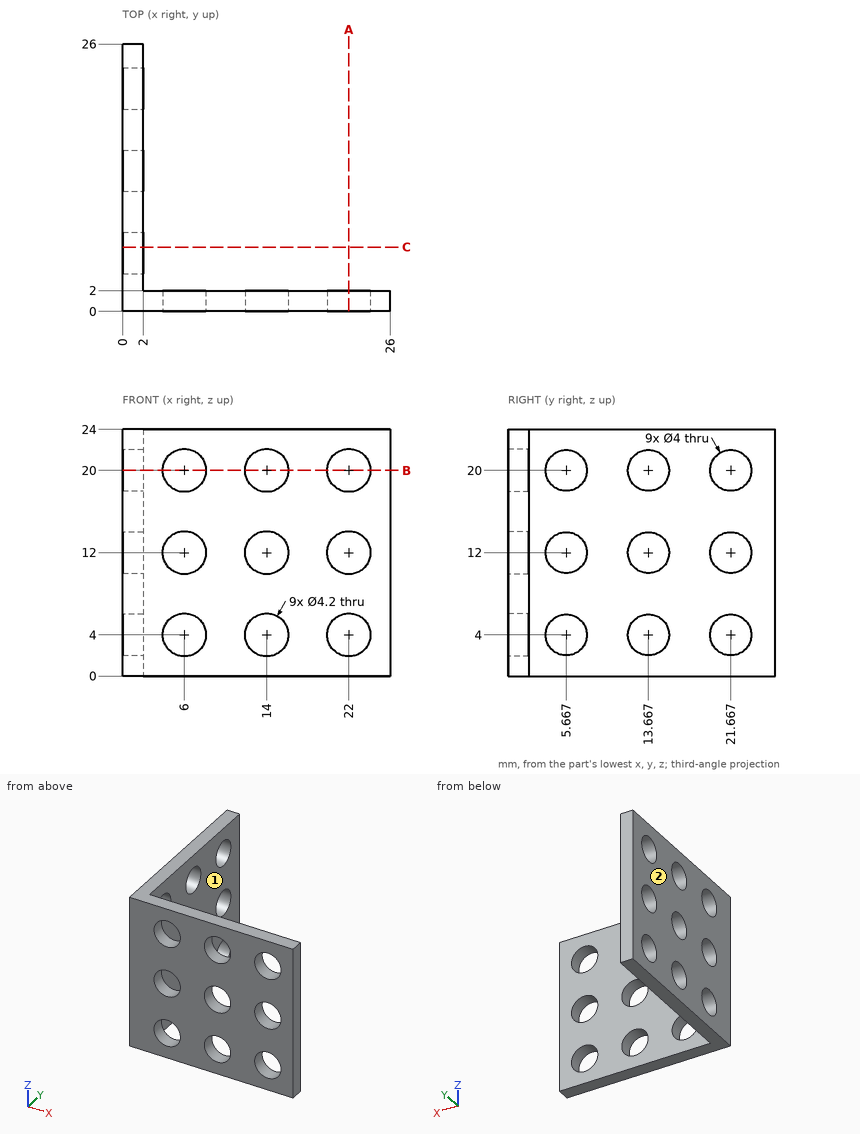
Part print with two shaded views. Sizes in mm from the minimum x, y, z corner. A direction names the side the tool comes from. Coordinates: 2 decimals unless noted, no trailing zeros. Loops run counter-clockwise (first coordinate to the right, second up) from the corner with the lowest first, then second, coordinate; pieces in that order, holes last. Notation, with made-up numbers: (-39.75, 68) -> (-1.75, 68) arc R35 cw to (-1.75, 102) -> close; hole circle Ø8 at (37.5, -18.5). An arc over 180 degrees is marked (long way). Answer as a JSON object with one key per item and string values.
Q1. Cut at A-A (x = 22). List the corners of the cut face in (y, z), and give its area (3 significant figures).
Report:
{"outline": "(0, 0) -> (2, 0) -> (2, 1.9) -> (0, 1.9) -> close; (0, 6.1) -> (2, 6.1) -> (2, 9.9) -> (0, 9.9) -> close; (0, 14.1) -> (2, 14.1) -> (2, 17.9) -> (0, 17.9) -> close; (0, 22.1) -> (2, 22.1) -> (2, 24) -> (0, 24) -> close", "area": "22.8 mm2"}
Q2. Flat gauge pins, fed straight in: P1, Ø4, axis at x = 6, z = 20, coming from the -Y side; P2, Ø5, axis at x = 8.5, z = 17, coming from the +Y side; P3, Ø5, axis at y = 21.67, z = 4, coming from the +X side. Where does each tip first touch, or does it go through?
Report:
{"P1": "passes through", "P2": "stops at y = 2", "P3": "stops at x = 2"}
Q3. Cut at B-B (z = 20). State how many separate pieces and enclosed holes the cut face has.
Report:
{"separate pieces": "7", "enclosed holes": "0"}
Q4. Probe probe 1 along Y at (x, z) = (1.1, 12); probe 2 along X at (y, z) = (0.55, 20); probe 3 along Y at (x, z) = (17.75, 22.5). List the from-to ranges inside material, lowest first.
Report:
{"probe 1": "y = 0 to 3.67, 7.67 to 11.67, 15.67 to 19.67, 23.67 to 26", "probe 2": "x = 0 to 3.9, 8.1 to 11.9, 16.1 to 19.9, 24.1 to 26", "probe 3": "y = 0 to 2"}
Q5. Cut at C-C (y = 6.25). List the corners of the cut face in (x, z).
Report:
{"outline": "(0, 0) -> (2, 0) -> (2, 2.09) -> (0, 2.09) -> close; (0, 5.91) -> (2, 5.91) -> (2, 10.09) -> (0, 10.09) -> close; (0, 13.91) -> (2, 13.91) -> (2, 18.09) -> (0, 18.09) -> close; (0, 21.91) -> (2, 21.91) -> (2, 24) -> (0, 24) -> close"}
Q6. 3-axis set-ups, long thin cutter, end or side, ignore diameter. For the marked faces 1 and 2: which of +Z, -Z, +X, -X, +Y, -Y reach the whole face in a straight line?
Report:
{"face 1": "+Z, -Z, +X, +Y", "face 2": "+Z, -Z, -X, +Y, -Y"}
